Verification items for this drawing (mm, ordinates from the low corner). A direction names the side the tool comes from. Coordinates: 2 decimals unless noted, no trailing zeros. Loops run counter-clockwise (first coordinate to the right, second up) from the corner with the lowest first, then second, coordinate; pieces in that order, holes last. Notation, with made-up numbers: (-29, 62.25) - (11, 62.25) arc R23 ccw to (11, 86.25) - close; hole circle Ø8 at (14.25, -19.75). An arc over 180 degrees is marked (long way). One line per item, written item: value. Start each with the question number.
(1) Draft check along Z on the marked faces 1, 2, 3 and 4. Enter one of: +Z half, -Z half, draft (parallel to the pull), parting line (faces both ways), or undercut.
(2) Section check C-C (y = 14). Record the boundary of the cut face in (x, z), plus the area to 3 significant figures.
(3) Section check A-A (z = 52.5). Record the boundary of the cut face in (x, y).
(4) Section check B-B (x = 52.5). Record the boundary of the cut face in (y, z).
(5) Thickness scan on probe 1 along X at (y, z) = (5.75, 52.5); probe 2 along X at (y, z) = (23.45, 52.5); probe 3 along Y at (x, z) = (93, 49.5). Record the ranges inside material, lowest first. Write a range as [from, to].
(6) Section check D-D (x = 93.5). Record the boundary of the cut face in (y, z).
(7) Gauge pin test, flat ends, axial feed: P1, Ø12, axis at x = 89.5, y = 14.5, coming from the +Z side; P2, Ø8, axis at y = 11, z = 16, coming from the -X side; P3, Ø1, axis at y = 8.5, z = 82, coming from the +X side. Record the tip position at first contact, or that the pin passes through.
(8) Set-up check for the marked faces 5 and 6: record each of +Z, -Z, +X, -X, +Y, -Y from which the full face is reachable in a straight line by a thin tool's end or side.
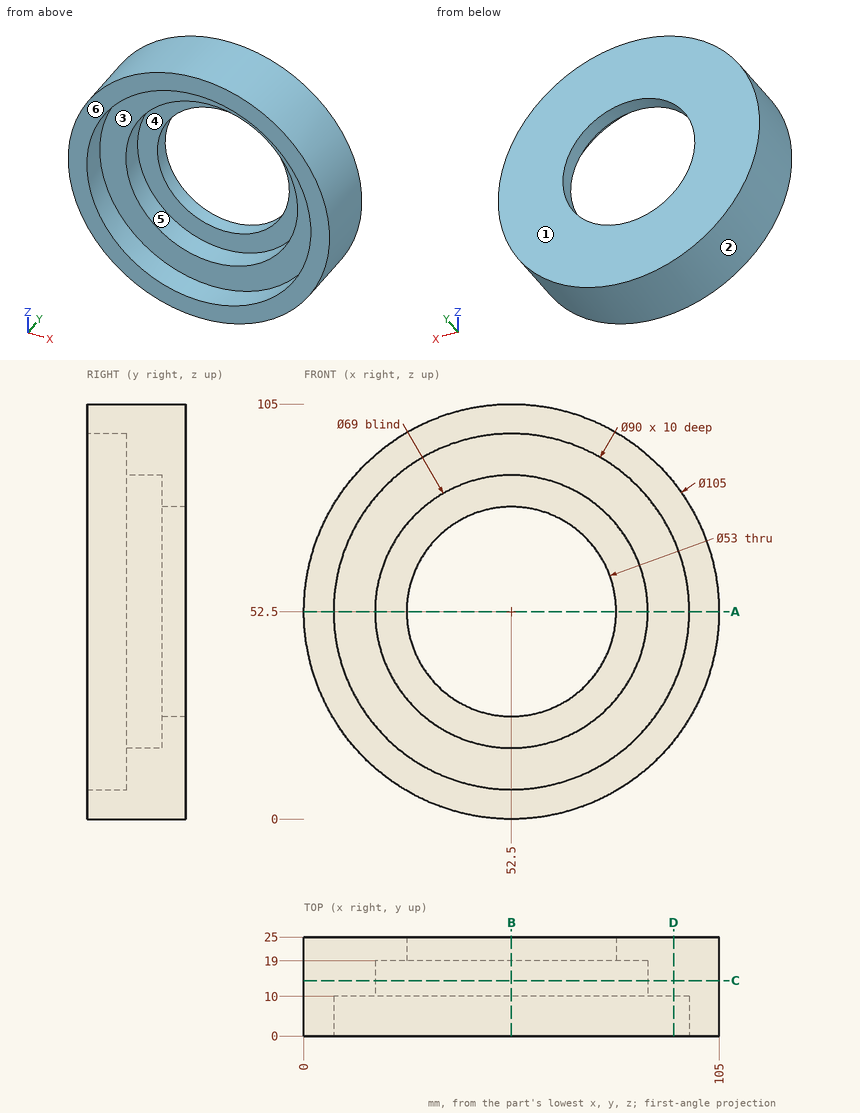
Responses:
1. face 1: draft
1. face 2: parting line
1. face 3: undercut
1. face 4: undercut
2. outline: circle Ø105 at (52.5, 52.5); hole circle Ø69 at (52.5, 52.5)
2. area: 4,920 mm²
3. outline: (0, 0) - (7.5, 0) - (7.5, 10) - (18, 10) - (18, 19) - (26, 19) - (26, 25) - (0, 25) - close; (79, 19) - (87, 19) - (87, 10) - (97.5, 10) - (97.5, 0) - (105, 0) - (105, 25) - (79, 25) - close
4. outline: (0, 0) - (25, 0) - (25, 26) - (19, 26) - (19, 18) - (10, 18) - (10, 7.5) - (0, 7.5) - close; (0, 97.5) - (10, 97.5) - (10, 87) - (19, 87) - (19, 79) - (25, 79) - (25, 105) - (0, 105) - close
5. probe 1: x = [0, 7.5], [97.5, 105]
5. probe 2: x = [0, 26], [79, 105]
5. probe 3: y = [10, 25]
6. outline: (0, 19.71) - (25, 19.71) - (25, 85.29) - (0, 85.29) - (0, 71.05) - (10, 71.05) - (10, 33.95) - (0, 33.95) - close
7. P1: stops at z = 94.87
7. P2: stops at x = 11.27
7. P3: stops at x = 96.26
8. face 5: -Y
8. face 6: +Z, -Z, +X, -X, -Y
